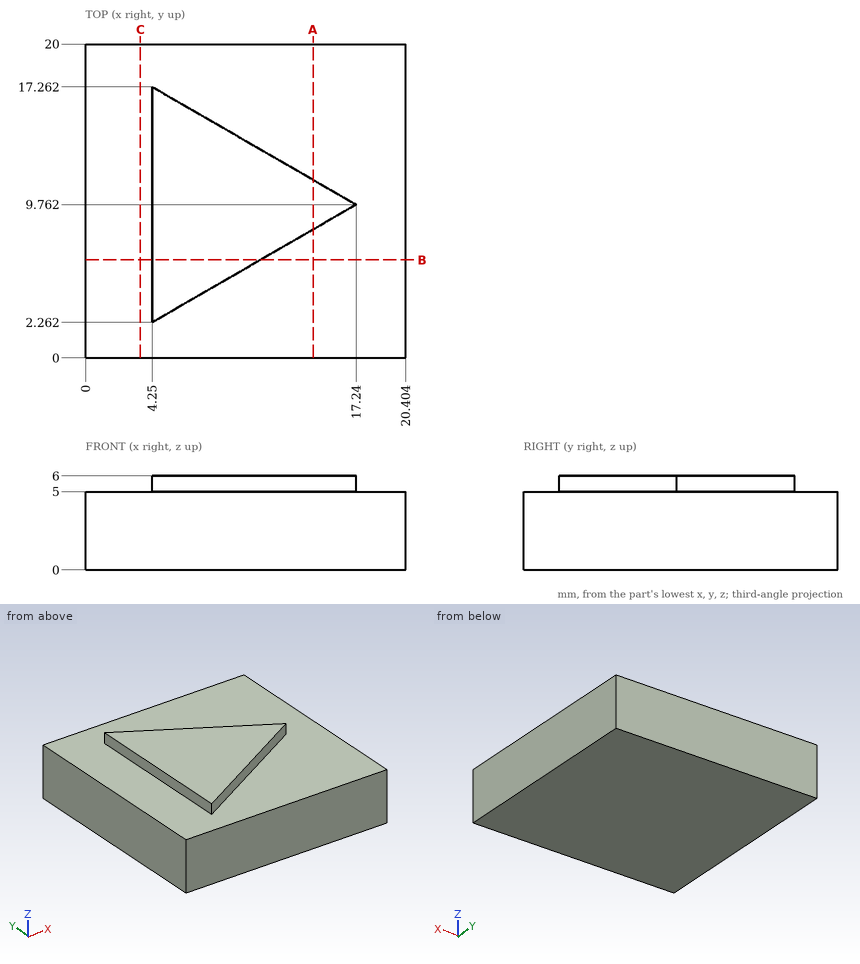
Design review of the part shown in the three views and the two pictorial views. Dimensions are in mm from the part's minimum x, y and z. Coordinates: 2 decimals unless noted, no trailing zeros. Loops run counter-clockwise (first coordinate to the right, second up) from the corner with the lowest first, then second, coordinate; pieces in that order, holes last.
Q1. For pin 1 (1.5 mm diameter, centred on y = 6, z = 4, fed in from -X); pin 2 (0.5 mm diameter, centred on y = 8.5, z = 5.5, fed in from -X), all flat-tipped, find the tip position at first contact; note any pin that passes through.
Reported:
pin 1: stops at x = 0
pin 2: stops at x = 4.25
Q2. We need section A-A on x = 14.5. State the section outline as (y, z) points (1 decimal).
Reported:
outline: (0, 0) - (20, 0) - (20, 5) - (11.3, 5) - (11.3, 6) - (8.2, 6) - (8.2, 5) - (0, 5) - close
Q3. We need section B-B on y = 6.25. State the section outline as (x, z) points, and give its area (3 significant figures).
Reported:
outline: (0, 0) - (20.4, 0) - (20.4, 5) - (11.16, 5) - (11.16, 6) - (4.25, 6) - (4.25, 5) - (0, 5) - close
area: 109 mm2
Q4. To check wall thickness, follow line 1 (Z direction, x = 17.5, y = 3). State the ranges of the line that lie inside material, in increasing order.
Reported:
line 1: z = 0 to 5
Q5. We need section C-C on x = 3.5. State the section outline as (y, z) points.
Reported:
outline: (0, 0) - (20, 0) - (20, 5) - (0, 5) - close
